Can you work these out from the drawing? Everything is in mm from the part's minimum corner. Coordinates: 2 decimals unless noted, no trailing zeros. Order: outer loops, then holes, each group sorted by start corner. A loop starts at its lowest first (then second) coordinate and runs counter-clockwise, first axis right, second up. Notation, with made-up numbers: (81.5, -2) - (130.5, -2) arc R15 ccw to (130.5, 10) - close; hole circle Ø8 at (0, 70.25). An arc over 180 degrees is marked (long way). One line per item, written item: value.
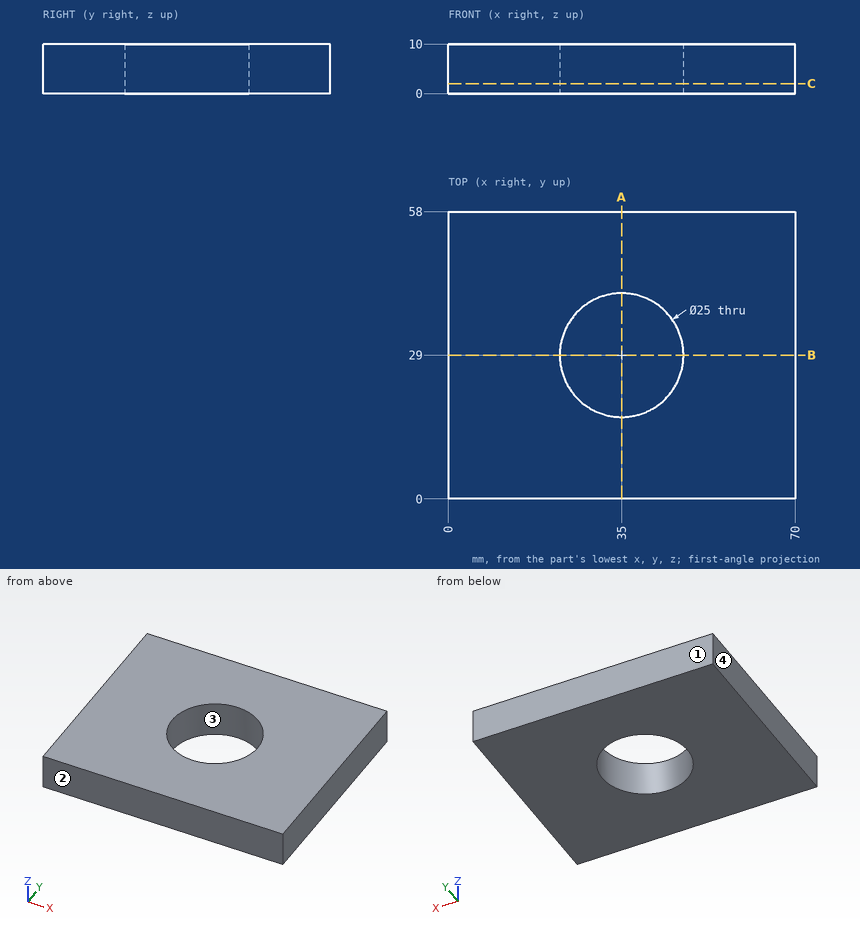
Item 1: Thinking about a two-plate mould opening in Y: for the marked faces 1, 2, 3 and 4, which applies, pulls with the +Y half, pulls with the -Y half, needs draft (parallel to the pull), parting line crosses it, or undercut?
Conclusion:
face 1: pulls with the +Y half
face 2: pulls with the -Y half
face 3: undercut
face 4: needs draft
Item 2: If I drill on probe 1 along Y at (x, z) = (35, 8); probe 2 along X at (y, z) = (28.5, 3); probe 3 along X at (y, z) = (32, 6), over which ranges is the centre line in solid material (lowest first)?
Conclusion:
probe 1: 0 to 16.5, 41.5 to 58
probe 2: 0 to 22.51, 47.49 to 70
probe 3: 0 to 22.87, 47.13 to 70
Item 3: I want a section at A-A on x = 35. Please give me the cut outline in (y, z).
Conclusion:
outline: (0, 0) - (16.5, 0) - (16.5, 10) - (0, 10) - close; (41.5, 0) - (58, 0) - (58, 10) - (41.5, 10) - close
Item 4: I want a section at B-B on y = 29. Please give me the cut outline in (x, z), then the cut area to 3 significant figures.
Conclusion:
outline: (0, 0) - (22.5, 0) - (22.5, 10) - (0, 10) - close; (47.5, 0) - (70, 0) - (70, 10) - (47.5, 10) - close
area: 450 mm²
Item 5: I want a section at C-C on z = 2. Please give me the cut outline in (x, y), then the cut area to 3 significant figures.
Conclusion:
outline: (0, 0) - (70, 0) - (70, 58) - (0, 58) - close; hole circle Ø25 at (35, 29)
area: 3,570 mm²
